Here's how the part is built. I have some questions about the finished solid (model axes, mm). Face numbers are marked on the shaded views. Coordinates: 2 decimals unless noted, no trailing zeros. Order: outer loops, then holes, each group sorted by start corner. A loop starts at its lowest first (then second) coordinate and runs counter-clockwise, first axis right, second up. Notation, with made-up numbers: (77, 87) - (121, 87) arc R24 ccw to (121, 115) - close; hole circle Ø3 at (75, 35). An arc over 180 degrees is marked (long way). Answer in a Markdown table with one row per item. Add a question column.
Item 1: If I drill on line 1 along X through (y, z) = (187.5, 0.45); line 2 along Z through (x, y) = (-29.5, -5); line 3 along Y through (x, z) = (-49, -268), over which ranges is the centre line in solid material (lowest first)? Write a range as from..to.
Item 2: I want a section at B-B (x = -21). Please give me the cut outline in (y, z), plus the area to 3 significant figures.
Item 3: Thinking about a two-plate mould opening in Z: for the marked faces 1 and 2, which applies, +Z half, -Z half, draft (parallel to the pull), parting line (faces both ways), or undercut?
Item 4: I want a section at D-D (z = -27). Please give me the cut outline in (x, y).
Item 5: I want a section at C-C (z = -70). Please give me the cut outline in (x, y), plus the area to 3 significant figures.
Item 6: Will these pins go through, and if not, where does the flat tip stop? pin 1 Ø1.3 at (x, z) = (-9.5, -52) entering from -Y; pin 2 Ø2.5 at (x, z) = (-25, -303) entering from +Y; pin 3 Ø7.5 at (y, z) = (180.5, -65) entering from -X.
Item 7: I want a section at A-A (y = 92.5). Please give me the cut outline in (x, z), plus the area to 3 significant figures.
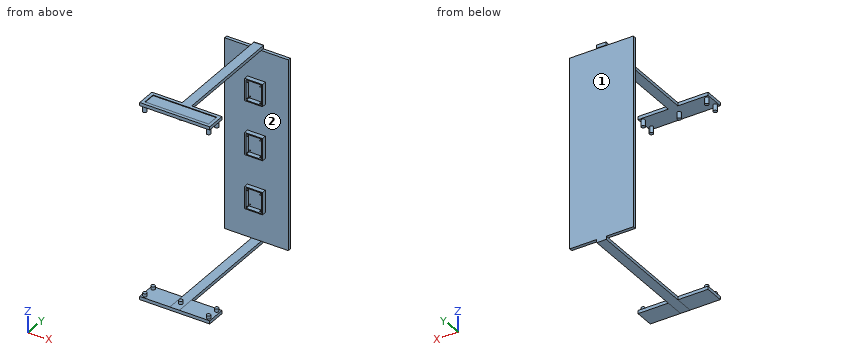
```python
from build123d import *

# Parameters (mm, degrees)
SKETCH2_W            = 110
SKETCH2_H            = 30
SKETCH2_W_2          = 100
SKETCH2_H_2          = 20
BOSS_EXTRUDE1_DEPTH  = 5
SKETCH3_R            = 2.446699787
CUT_EXTRUDE3_DEPTH   = 15
SKETCH3_10_W         = 15
SKETCH3_10_H         = 5
SKETCH3_10_R         = 2.446699787
BOSS_EXTRUDE4_DEPTH  = 175
SKETCH12_W           = 100
SKETCH12_H           = 20
BOSS_EXTRUDE12_DEPTH = 1
SKETCH5_W            = 15
SKETCH5_H            = 5
BOSS_EXTRUDE13_DEPTH = 300
SKETCH13_R           = 2
CUT_EXTRUDE10_DEPTH  = 301
BOSS_EXTRUDE16_DEPTH = 205
SKETCH22_R           = 3
BOSS_EXTRUDE20_DEPTH = 10
SKETCH26_W           = 110
SKETCH26_H           = 30
BOSS_EXTRUDE22_DEPTH = 5
SKETCH27_R           = 3
BOSS_EXTRUDE23_DEPTH = 5
SKETCH28_W           = 28
SKETCH28_H           = 35
SKETCH28_W_2         = 25
SKETCH28_H_2         = 32
BOSS_EXTRUDE26_DEPTH = 7
BOSS_EXTRUDE28_DEPTH = 42.5
BOSS_EXTRUDE29_DEPTH = 57.5
BOSS_EXTRUDE30_DEPTH = 1
SKETCH30_R           = 0.6
BOSS_EXTRUDE32_DEPTH = 7.5
BOSS_EXTRUDE34_DEPTH = 3


with BuildPart() as part:
    # Sketch2 → Boss-Extrude1 (new body)
    with BuildSketch(Plane.XY):
        Rectangle(SKETCH2_W, SKETCH2_H)
        Rectangle(SKETCH2_W_2, SKETCH2_H_2, mode=Mode.SUBTRACT)
    extrude(amount=BOSS_EXTRUDE1_DEPTH)

    # Sketch3 → Cut-Extrude3 (cut)
    with BuildSketch(Plane(origin=(0, 15, 0), x_dir=(1, 0, 0), z_dir=(0, 1, 0))):
        with Locations(Location((4.931689359, -2.5, 0), (0, 0, 180))):
            Circle(SKETCH3_R)
        with Locations(Location((-0.068310641, -2.5, 0), (0, 0, 180))):
            Circle(SKETCH3_R)
        with Locations(Location((-5.068310641, -2.5, 0), (0, 0, 180))):
            Circle(SKETCH3_R)
    extrude(amount=-CUT_EXTRUDE3_DEPTH, mode=Mode.SUBTRACT)

    # Sketch3<10> → Boss-Extrude4 (add)
    with BuildSketch(Plane(origin=(0, 15, 0), x_dir=(1, 0, 0), z_dir=(0, 1, 0))):
        with Locations((-0.068310641, -2.5)):
            Rectangle(SKETCH3_10_W, SKETCH3_10_H)
        with Locations(Location((-0.068310641, -2.5, 0), (0, 0, 180))):
            Circle(SKETCH3_10_R, mode=Mode.SUBTRACT)
        with Locations(Location((4.931689359, -2.5, 0), (0, 0, 180))):
            Circle(SKETCH3_10_R, mode=Mode.SUBTRACT)
        with Locations(Location((-5.068310641, -2.5, 0), (0, 0, 180))):
            Circle(SKETCH3_10_R, mode=Mode.SUBTRACT)
    extrude(amount=BOSS_EXTRUDE4_DEPTH)

    # Sketch12 → Boss-Extrude12 (add)
    with BuildSketch(Plane(origin=(0, 0, 0), x_dir=(-1, 0, 0), z_dir=(0, 0, -1))):
        Rectangle(SKETCH12_W, SKETCH12_H)
    extrude(amount=-BOSS_EXTRUDE12_DEPTH)

    # Sketch5 → Boss-Extrude13 (add)
    with BuildSketch(Plane(origin=(0, 0, 0), x_dir=(-1, 0, 0), z_dir=(0, 0, -1))):
        with Locations((0.068310641, 187.5)):
            Rectangle(SKETCH5_W, SKETCH5_H)
    extrude(amount=BOSS_EXTRUDE13_DEPTH)

    # Sketch13 → Cut-Extrude10 (cut)
    with BuildSketch(Plane(origin=(0, 0, -300), x_dir=(-1, 0, 0), z_dir=(0, 0, -1))):
        with Locations((-4.931689359, 187.5)):
            Circle(SKETCH13_R)
        with Locations((0.068310641, 187.5)):
            Circle(SKETCH13_R)
        with Locations((5.068310641, 187.5)):
            Circle(SKETCH13_R)
    extrude(amount=-CUT_EXTRUDE10_DEPTH, mode=Mode.SUBTRACT)

    # 3DSketch1 → Boss-Extrude16 (add)
    with BuildSketch(Plane(origin=(-7.568310641, 190, -300), x_dir=(0.9486832980505138, 0, -0.3162277660168382), z_dir=(0, -1, 0))):
        Polygon((0, 0), (14.230249471, 4.74341649), (15.811388301, 0), (1.58113883, -4.74341649), align=None)
    extrude(amount=BOSS_EXTRUDE16_DEPTH)

    # Sketch22 → Boss-Extrude20 (add)
    with BuildSketch(Plane(origin=(0, 0, 0), x_dir=(-1, 0, 0), z_dir=(0, 0, -1))):
        with BuildLine():
            ThreePointArc((-50, -7), (-52.121320344, -12.121320344), (-47, -10))
            Line((-47, -10), (-50, -10))
            Line((-50, -10), (-50, -7))
        make_face()
        with BuildLine():
            Line((-50, -10), (-47, -10))
            ThreePointArc((-47, -10), (-47.878679656, -7.878679656), (-50, -7))
            Line((-50, -7), (-50, -10))
        make_face()
        with Locations(Location((0, 0, 0), (0, 0, 180))):
            Circle(SKETCH22_R)
        with Locations(Location((-50, 10, 0), (0, 0, 180))):
            Circle(SKETCH22_R)
        with Locations(Location((50, 10, 0), (0, 0, 180))):
            Circle(SKETCH22_R)
        with Locations(Location((50, -10, 0), (0, 0, 180))):
            Circle(SKETCH22_R)
    extrude(amount=BOSS_EXTRUDE20_DEPTH)

    # Sketch26 → Boss-Extrude22 (add)
    with BuildSketch(Plane(origin=(0, 0, -305), x_dir=(-1, 0, 0), z_dir=(0, 0, -1))):
        Rectangle(SKETCH26_W, SKETCH26_H)
    extrude(amount=-BOSS_EXTRUDE22_DEPTH)

    # Sketch27 → Boss-Extrude23 (add)
    with BuildSketch(Plane.XY.offset(-300)):
        Circle(SKETCH27_R)
        with Locations((-50, 10)):
            Circle(SKETCH27_R)
        with Locations((-50, -10)):
            Circle(SKETCH27_R)
        with Locations((50, 10)):
            Circle(SKETCH27_R)
        with Locations((50, -10)):
            Circle(SKETCH27_R)
    extrude(amount=BOSS_EXTRUDE23_DEPTH)

    # Sketch28 → Boss-Extrude26 (add)
    with BuildSketch(Plane.XZ.offset(-185)):
        with Locations((-0.068310641, -150)):
            Rectangle(SKETCH28_W, SKETCH28_H)
        with Locations((0.231689359, -150)):
            Rectangle(SKETCH28_W_2, SKETCH28_H_2, mode=Mode.SUBTRACT)
        with Locations((-0.068310641, -235)):
            Rectangle(SKETCH28_W, SKETCH28_H)
        with Locations((0.231689359, -235)):
            Rectangle(SKETCH28_W_2, SKETCH28_H_2, mode=Mode.SUBTRACT)
        with Locations((-0.068310641, -65)):
            Rectangle(SKETCH28_W, SKETCH28_H)
        with Locations((0.231689359, -65)):
            Rectangle(SKETCH28_W_2, SKETCH28_H_2, mode=Mode.SUBTRACT)
    extrude(amount=BOSS_EXTRUDE26_DEPTH)

    # 3DSketch4 → Boss-Extrude28 (add)
    with BuildSketch(Plane(origin=(-7.568310641, 185, -300), x_dir=(0, 0.01666435233399335, 0.9998611400396), z_dir=(-1, 0, 0))):
        Polygon((0, 0), (0.083321762, 4.9993057), (300.041663774, 0), (299.958342012, -4.9993057), align=None)
    extrude(amount=BOSS_EXTRUDE28_DEPTH)

    # 3DSketch4<4> → Boss-Extrude29 (add)
    with BuildSketch(Plane(origin=(-7.568310641, 185, -300), x_dir=(0, 0.01666435233399335, 0.9998611400396), z_dir=(-1, 0, 0))):
        Polygon((0, 0), (0.083321762, 4.9993057), (300.041663774, 0), (299.958342012, -4.9993057), align=None)
    extrude(amount=-BOSS_EXTRUDE29_DEPTH)

    # 3DSketch5 → Boss-Extrude30 (add)
    with BuildSketch(Plane(origin=(-7.568310641, 190, 5), x_dir=(0.9486832980505139, 0, -0.31622776601683783), z_dir=(0, 1, 0))):
        Polygon((0, 0), (1.58113883, 4.74341649), (15.811388301, 0), (14.230249471, -4.74341649), align=None)
    extrude(amount=BOSS_EXTRUDE30_DEPTH)

    # Sketch30 → Boss-Extrude32 (add)
    with BuildSketch(Plane.XZ.offset(-185)):
        with Locations(Location((-9.923310641, -248.1916, 0), (0, 0, 90))):
            Circle(SKETCH30_R)
        with Locations(Location((10.386689359, -248.1916, 0), (0, 0, 90))):
            Circle(SKETCH30_R)
        with Locations(Location((-9.923310641, -222.0016, 0), (0, 0, 90))):
            Circle(SKETCH30_R)
        with Locations(Location((10.386689359, -222.0016, 0), (0, 0, 90))):
            Circle(SKETCH30_R)
        with Locations(Location((10.462158109, -163.095, 0), (0, 0, 90))):
            Circle(SKETCH30_R)
        with Locations(Location((-9.847841891, -163.095, 0), (0, 0, 90))):
            Circle(SKETCH30_R)
        with Locations(Location((-9.847841891, -136.905, 0), (0, 0, 90))):
            Circle(SKETCH30_R)
        with Locations(Location((10.462158109, -136.905, 0), (0, 0, 90))):
            Circle(SKETCH30_R)
        with Locations(Location((10.462158109, -51.905, 0), (0, 0, 90))):
            Circle(SKETCH30_R)
        with Locations(Location((-9.847841891, -51.905, 0), (0, 0, 90))):
            Circle(SKETCH30_R)
        with Locations(Location((-9.847841891, -78.095, 0), (0, 0, 90))):
            Circle(SKETCH30_R)
        with Locations(Location((10.462158109, -78.095, 0), (0, 0, 90))):
            Circle(SKETCH30_R)
    extrude(amount=BOSS_EXTRUDE32_DEPTH)

    # 3DSketch6 → Boss-Extrude34 (add)
    with BuildSketch(Plane(origin=(-50, 10, 1), x_dir=(0.9805806756909201, -0.19611613513818413, 0), z_dir=(0, 0, 1))):
        Polygon((0, 0), (98.058067569, 19.611613514), (101.980390272, 0), (3.922322703, -19.611613514), align=None)
    extrude(amount=BOSS_EXTRUDE34_DEPTH)


solid = part.part
```
Values follow:
| question | item | result |
|---|---|---|
| 1 | line 1 | x = -7.57..-7.07, -3.07..-2.07, 1.93..2.93, 6.93..7.43 |
| 1 | line 2 | z = -305..-300, 0..4 |
| 1 | line 3 | y = 185..190 |
| 2 | outline | (-15, -305) - (15, -305) - (15, -300) - (-15, -300) - close; (-15, 0) - (15, 0) - (15, 5) - (10, 5) - (10, 4) - (-10, 4) - (-10, 5) - (-15, 5) - close; (185, -300) - (190, -300) - (190, 0) - (185, 0) - close |
| 2 | area | 1,780 mm^2 |
| 3 | face 1 | draft |
| 3 | face 2 | undercut |
| 4 | outline | (-50.07, 185) - (49.93, 185) - (49.93, 190) - (-50.07, 190) - close |
| 5 | outline | (-50.07, 185) - (-14.07, 185) - (-14.07, 178) - (-12.27, 178) - (-12.27, 185) - (12.73, 185) - (12.73, 178) - (13.93, 178) - (13.93, 185) - (49.93, 185) - (49.93, 190) - (-50.07, 190) - close |
| 5 | area | 521 mm^2 |
| 6 | pin 1 | stops at y = 177.5 |
| 6 | pin 2 | stops at y = 15 |
| 6 | pin 3 | stops at x = -14.07 |
| 7 | outline | (-7.57, -305) - (7.43, -305) - (7.43, -300) - (-7.57, -300) - close; (-7.57, 0) - (7.43, 0) - (7.43, 5) - (-7.57, 5) - close; hole circle Ø4.89 at (-5.07, 2.5); hole circle Ø4.89 at (-0.07, 2.5); hole circle Ø4.89 at (4.93, 2.5) |
| 7 | area | 93.6 mm^2 |
